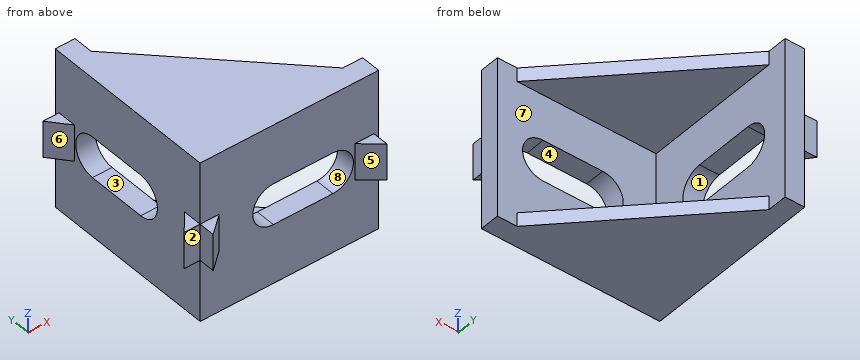
Autodesk Inventor part; units mm, degrees
ref_plane "Arbeitsebene1" through (4.3, 4.3, 0) normal (-0.7071, 0.7071, 0) x (0, 0, 1)
ref_plane "YZ Plane" through (0, 0, 0) normal (1, 0, 0) x (0, 1, 0)
ref_plane "XY Plane" through (0, 0, 0) normal (0, 0, 1) x (1, 0, 0)
sketch "Skizze1" plane through (0, 0, 0) normal (0, 0, 1) x (1, 0, 0)
  line L0 (-12, 0) -> (47.5, 0)
  line L1 (0, 47.5) -> (0, -12)
  line L2 (39, 0) -> (39, 4.3)
  line L3 (39, 4.3) -> (34.6772, 4.3)
  line L4 (34.6772, 4.3) -> (4.3, 34.6772)
  line L5 (4.3, 34.6772) -> (4.3, 39)
  line L6 (4.3, 39) -> (0, 39)
  line L7 (0, 39) -> (0, 0)
  line L8 (0, 0) -> (39, 0)
  line L9 (34.6772, 4.3) -> (4.3, 4.3)
  line L10 (4.3, 4.3) -> (4.3, 34.6772)
  line L11 (0, 38) -> (-3.5, 38)
  line L12 (-3.5, 38) -> (0, 33.8289)
  line L13 (0, 4.1711) -> (-3.5, 0)
  line L14 (0, 0) -> (-3.5, 0)
  line L15 (0, 0) -> (0, -3.5)
  line L16 (0, -3.5) -> (4.1711, 0)
  line L17 (38, 0) -> (38, -3.5)
  line L18 (38, -3.5) -> (33.8289, 0)
  dimension "d0" = 39
  dimension "d1" = 39
  dimension "d2" = 4.3
  dimension "d3" = 4.3
  dimension "d4" = 45
  dimension "d7" = 40
  dimension "d8" = 40
  dimension "d9" = 40
  dimension "d10" = 40
  dimension "d11" = 3.5
  dimension "d12" = 3.5
  dimension "d13" = 3.5
  dimension "d14" = 3.5
  dimension "d15" = 1
  dimension "d16" = 1
extrude "Extrusion1" add sketch "Skizze1" along normal mid plane 35 contours L1 L6 L5 L10 L9 L3 L2 L0
extrude "Extrusion2" add sketch "Skizze1" along normal mid plane 8 contours L13 L1 L0 | L0 L16 L1 | L12 L11 L1 | L0 L17 L18
extrude "Extrusion3" add sketch "Skizze1" against normal blind 3 from surface at 17.5 contours L4 L9 L10
extrude "Extrusion4" add sketch "Skizze1" along normal blind 3 from surface at -17.5 contours L4 L9 L10
sketch "Skizze2" plane through (4.3, 39, 17.5) normal (1, 0, 0) x (0, 0, -1)
  line L0 (0, 0) -> (35, 0)
  line L1 (0, -4.3228) -> (0, 0)
  line L2 (0, -4.3228) -> (3, -4.3228)
  line L3 (3, -34.7) -> (3, -4.3228)
  line L4 (32, -34.7) -> (3, -34.7)
  line L5 (32, -4.3228) -> (32, -34.7)
  line L6 (32, -4.3228) -> (35, -4.3228)
  line L7 (35, 0) -> (35, -4.3228)
  line L8 (32, -4.3228) -> (35, -4.3228) construction
  line L9 (0, -4.3228) -> (3, -4.3228) construction
  line L10 (32, -34.7) -> (3, -34.7) construction
  line L11 (17.5, -23) -> (17.5, -10) construction
  line L12 (22, -23) -> (22, -10)
  line L13 (13, -10) -> (13, -23)
  arc A0 (13, -23) -> (22, -23) centre (17.5, -23) ccw
  arc A1 (22, -10) -> (13, -10) centre (17.5, -10) ccw
  line L14 (35, 0) -> (0, 0) construction
  line L15 (17.5, 0) -> (17.5, -49.0584) construction
  point P0 (17.5, -39)
  point P1 (17.5, -16.5)
  point P2 (17.5, -27.5)
  point P3 (17.5, -5.5)
  dimension "d23" = 6.5
  dimension "d24" = 9
  dimension "d25" = 22
  dimension "d26" = 5.5
extrude "Extrusion5" cut sketch "Skizze2" against normal blind 5 contours A0 L13 A1 L12
ref_plane "Arbeitsebene1" through (4.3, 4.3, 0) normal (-0.7071, 0.7071, 0) x (0, 0, 1)
mirror "Spiegeln1" about plane through (4.3, 4.3, 0) normal (-0.7071, 0.7071, 0) of "Extrusion5"
equation "\"d12\" = d11"
equation "\"d13\" = d11"
equation "\"d14\" = d11"
properties part number "Bracket - Cast 90 deg corner 4040"
Work out the finished part from the listing and answer in its coordinate system (mm). Face numbers are marked on the shaded views. A direction names the side the tool comes from. Round coordinates to 2 decimals unless told otherwise and drop trailing zeros. Loops run counter-clockwise (first coordinate to the right, second up) from the corner with the lowest first, then second, coordinate; pieces in that order, holes last. Notation, with made-up numbers: M -7.75,61 L 40.25,61 A31 ccw 40.25,100 Z; hole C 35.25,17.25 d11. An arc over 180 degrees is marked long. Use CSV: the item, a comma, the result in double quotes.
Q1. Section C-C, the plane x = 32 is taken. Determine the outline of the cut face in (y, z), then the cut area to 3 significant figures.
Determined:
outline,"M 0,-17.5 L 6.98,-17.5 L 6.98,-14.5 L 4.3,-14.5 L 4.3,-3.35 L 0,-3.35 Z; M 0,3.35 L 4.3,3.35 L 4.3,14.5 L 6.98,14.5 L 6.98,17.5 L 0,17.5 Z"
area,"138 mm2"
Q2. Section D-D, the plane z = 5.5 is taken. Determine the outline of the cut face in (x, y).
Determined:
outline,"M 0,0 L 39,0 L 39,4.3 L 4.3,4.3 L 4.3,39 L 0,39 Z"
Q3. Consider L1, parallel to Z at x = 19.5, y = 4.5; L2, parallel to X at y = 4, z = -5; L3, parallel to X at y = 26, z = -11.5. Determine where each line is inside the solid, lowest interval first.
Determined:
L1,"-17.5 to -14.5, 14.5 to 17.5"
L2,"0 to 39"
L3,"0 to 4.3"
Q4. A tool of negligible diameter and unlimited length cuts with its end or side. For the marked faces 5, 6, 7 and 8, from which of +Z, -Z, +X, -X, +Y, -Y can it reach the whole face along a straight path? Write none if from no direction.
Determined:
face 5,"+Z, -Z, -Y"
face 6,"+Z, -Z, -X"
face 7,"+X, +Y"
face 8,"+Y, -Y"
Q5. The mould has two halves that part along Y. Classify the marked faces 1, 2, 3 and 4: pulls with the +Y half, pulls with the -Y half, needs draft (parallel to the pull), parting line crosses it, or undercut.
Determined:
face 1,"undercut"
face 2,"pulls with the -Y half"
face 3,"undercut"
face 4,"needs draft"
Q6. Each of these flat-tipped pins is pushed along its axis until it touches: pin 1 (1.1 mm diameter, centred on x = -1.5, y = 36, fed in from -Z); pin 2 (5 mm diameter, centred on x = 30.5, z = 2, fed in from -Y); pin 3 (8 mm diameter, centred on y = 20.5, z = 7, fed in from +X); pin 4 (1.1 mm diameter, centred on x = 35.5, y = -2.5, fed in from +Z). Where does it stop, or does it pass through?
Determined:
pin 1,"z = -4"
pin 2,"y = 0"
pin 3,"x = 4.3"
pin 4,"through"
Q7. Section B-B, the plane y = 18.5 is taken. Determine the outline of the cut face in (x, z), then the cut area to 3 significant figures.
Determined:
outline,"M 0,-17.5 L 20.48,-17.5 L 20.48,-14.5 L 4.3,-14.5 L 4.3,-4.5 L 0,-4.5 Z; M 0,4.5 L 4.3,4.5 L 4.3,14.5 L 20.48,14.5 L 20.48,17.5 L 0,17.5 Z"
area,"209 mm2"
Q8. Section A-A, the plane z = 0 is taken. Determine the outline of the cut face in (x, y).
Determined:
outline,"M -3.5,0 L 0,0 L 0,-3.5 L 4.17,0 L 11.5,0 L 11.5,4.3 L 4.3,4.3 L 4.3,11.5 L 0,11.5 L 0,4.17 Z; M -3.5,38 L 0,33.83 L 0,33.5 L 4.3,33.5 L 4.3,39 L 0,39 L 0,38 Z; M 33.5,0 L 33.83,0 L 38,-3.5 L 38,0 L 39,0 L 39,4.3 L 33.5,4.3 Z"
